Source: CAD feature listing. Evaluate the final solid. Frame: model axes, mm. A direction names the side the tool comes from. Coordinates: 2 decimals unless noted, no trailing zeros. Order: outer loops, then holes, each group sorted by start corner. A loop starts at its lowest first (then second) coordinate and runs counter-clockwise, first axis right, second up. Notation, with made-up numbers: (-26, 53) -> (-1, 53) arc R27 cw to (-1, 88) -> close; hole circle Ø2 at (-12, 71). An arc over 180 degrees is marked (long way). Write each question's results on one line, items separated by ' | '. Start each with the question number.
from build123d import *

# Parameters (mm, degrees)
F1_DEPTH  = 50
F3_DEPTH  = 40
F4_W      = 10
F4_H      = 10
F5_DEPTH  = 40
F7_DEPTH  = 10
F8_W      = 40
F8_H      = 30
F9_DEPTH  = 40
F11_DEPTH = 25
F12_W     = 30
F12_H     = 30
F13_DEPTH = 10
F15_DEPTH = 10


with BuildPart() as f1:
    # F0 (on Front) → F1 (new body)
    with BuildSketch(Plane.XZ):
        Polygon((0, 30), (0, 0), (60, 0), (60, 50), (50, 50), (50, 20), (20, 20), (20, 30), align=None)
    extrude(amount=F1_DEPTH)

    # F2 (on face) → F3 (cut)
    with BuildSketch(Plane.XZ.offset(50)):
        Polygon((10, 20), (10, 10), (60, 10), (60, 20), (50, 20), (20, 20), align=None)
    extrude(amount=-F3_DEPTH, mode=Mode.SUBTRACT)

    # F4 (on face) → F5 (cut)
    with BuildSketch(Plane.XZ.offset(50)):
        with Locations((15, 25)):
            Rectangle(F4_W, F4_H)
    extrude(amount=-F5_DEPTH, mode=Mode.SUBTRACT)

    # F6 (on face) → F7 (cut)
    with BuildSketch(Plane(origin=(0, 0, 0), x_dir=(0, -1, 0), z_dir=(-1, 0, 0))):
        Polygon((0, 30), (50, 10), (50, 30), align=None)
    extrude(amount=-F7_DEPTH, mode=Mode.SUBTRACT)

    # F8 (on face) → F9 (cut)
    with BuildSketch(Plane.YZ.offset(60)):
        with Locations((-30, 35)):
            Rectangle(F8_W, F8_H)
    extrude(amount=-F9_DEPTH, mode=Mode.SUBTRACT)

    # F10 (on face) → F11 (cut)
    with BuildSketch(Plane.XZ.offset(10)):
        with BuildLine():
            ThreePointArc((50, 50), (57.0710678119, 47.0710678119), (60, 40))
            Line((60, 40), (60, 50))
            Line((60, 50), (50, 50))
        make_face()
    extrude(amount=-F11_DEPTH, mode=Mode.SUBTRACT)

    # F12 (on face) → F13 (cut)
    with BuildSketch(Plane.XY.offset(10)):
        with Locations((45, -35)):
            Rectangle(F12_W, F12_H)
    extrude(amount=-F13_DEPTH, mode=Mode.SUBTRACT)

    # F14 (on face) → F15 (cut)
    with BuildSketch(Plane.XY.offset(10)):
        with BuildLine():
            ThreePointArc((60, -10), (57.0710678119, -17.0710678119), (50, -20))
            Line((50, -20), (60, -20))
            Line((60, -20), (60, -10))
        make_face()
        with BuildLine():
            Line((30, -50), (30, -40.9943062672))
            ThreePointArc((30, -40.9943062672), (28.2651766354, -46.407029811), (23.8608885556, -50))
            Line((23.8608885556, -50), (30, -50))
        make_face()
    extrude(amount=-F15_DEPTH, mode=Mode.SUBTRACT)


solid = f1.part
(1) Section C-C on y = -33. Return the cut outline in (x, z).
(2) Draft query along X for faces 1 (the cylindrical face through (57.15, -16.99, 5.07)), 2 (the flat face through (15, -5, 30)), 3 (the flat face through (50, -5, 35)). Return one class per face: released by +X, released by -X, zero draft, split by the parting line, or undercut.
(3) Line query: L1, parallel to Z at x = 10.5, y = -21.5; L2, parallel to X at y = -35, z = 8. Output: solid intervals per line, ascending.
(4) Reachability of faces 4 (the flat face through (35, -5, 20)), 5 (the flat face through (23, -19, 0)), 6 (the flat face through (5, -25, 20)), 7 (the flat face through (40, -20, 5)), 8 (the flat face through (41, -10, 16)) from +Z, -Z, +X, -X, +Y, -Y: full face, straight path, thin tool, end or side. Return the list, or none.
(5) Section D-D on x = 8.5. Return the cut outline in (y, z).
(6) Section B-B on z = 8.5. Return the cut outline in (x, y).
(7) First-contact query: P1, Ø6, axis at x = 12, z = 16, coming from the +Y side; P2, Ø8, axis at y = -26.5, z = 6.5, coming from the +X side; P3, Ø5, axis at y = -36.5, z = 16.5, coming from the +X side; P4, Ø3, axis at x = 12.5, y = -5.5, coming from the +Z side. Flat tips, straight axial feed; report the tip coordinate or a pass-through.
(8) Section A-A on x = 18.5. Return the cut outline in (y, z).
Results list:
1) outline: (0, 0) -> (30, 0) -> (30, 10) -> (10, 10) -> (10, 16.8) -> (0, 16.8) -> close
2) face 1: released by +X | face 2: zero draft | face 3: undercut
3) L1: z = 0 to 10 | L2: x = 0 to 30
4) face 4: +Z, +Y, -Y | face 5: -Z, +X, -X, +Y, -Y | face 6: +Z, -X, -Y | face 7: +Z, -Z, +X, -Y | face 8: +Z, +X, -Y
5) outline: (-50, 0) -> (0, 0) -> (0, 30) -> (-50, 10) -> close
6) outline: (0, -50) -> (23.86, -50) arc R10 ccw to (30, -40.99) -> (30, -20) -> (50, -20) arc R10 ccw to (60, -10) -> (60, 0) -> (0, 0) -> close
7) P1: stops at y = 0 | P2: stops at x = 30 | P3: stops at x = 10 | P4: stops at z = 30
8) outline: (-50, 0) -> (0, 0) -> (0, 30) -> (-10, 30) -> (-10, 10) -> (-50, 10) -> close
